from build123d import *

# Parameters (mm, degrees)
SKETCH1_W           = 28
SKETCH1_H           = 25
BOSS_EXTRUDE1_DEPTH = 2
SKETCH2_R           = 0.45
CUT_EXTRUDE1_DEPTH  = 10
SKETCH3_R           = 0.4
CUT_EXTRUDE2_DEPTH  = 2.5


with BuildPart() as part:
    # Sketch1 → Boss-Extrude1 (new body)
    with BuildSketch(Plane(origin=(0, 0, 0), x_dir=(1, 0, 0), z_dir=(0, 1, 0))):
        Rectangle(SKETCH1_W, SKETCH1_H)
    extrude(amount=BOSS_EXTRUDE1_DEPTH)

    # Sketch2 → Cut-Extrude1 (cut)
    with BuildSketch(Plane(origin=(0, 0, 0), x_dir=(1, 0, 0), z_dir=(0, 1, 0))):
        with Locations(Location((-9.52, -5.2, 0), (0, 0, 90))):
            Circle(SKETCH2_R)
        with Locations(Location((-9.52, -9.7, 0), (0, 0, 90))):
            Circle(SKETCH2_R)
    extrude(amount=CUT_EXTRUDE1_DEPTH, mode=Mode.SUBTRACT)

    # Sketch3 → Cut-Extrude2 (cut)
    with BuildSketch(Plane(origin=(0, 0, 0), x_dir=(1, 0, 0), z_dir=(0, 1, 0))):
        with Locations(Location((-11.13, 6.6, 0), (0, 0, 90))):
            Circle(SKETCH3_R)
        with Locations(Location((-11.13, 8.6, 0), (0, 0, 90))):
            Circle(SKETCH3_R)
        with Locations(Location((-11.13, 4.6, 0), (0, 0, 90))):
            Circle(SKETCH3_R)
    extrude(amount=CUT_EXTRUDE2_DEPTH, mode=Mode.SUBTRACT)


solid = part.part
Check sheet for the modelled part. Datum: model origin and axes. Units: mm. Round coordinates to 2 decimals unless told otherwise and drop trailing zeros. Write each loop counter-clockwise with the first axis right and the second up, starting at its lowest first coordinate (ties: lowest second). Pieces come first, ordered by that corner, then holes. Notation, with made-up numbers: (-9, 5.5) - (25, 5.5) arc R12 ccw to (25, 13.5) - close; hole circle Ø1 at (-3, -3.5). An arc over 180 degrees is marked (long way). Return JSON: item names as keys, results as strings.
Q1. Depth check by flat-ended pin: P1, Ø6, axis at x = -0.5, z = 7.5, coming from the -Y side. Enter the tip coordinate at first touch or a pass-through.
Returned:
{"P1": "stops at y = 0"}
Q2. Scan lines: L1, parallel to Z at x = -11.13, y = 1.65; L2, parallel to X at y = 0.95, z = 9.7; L3, parallel to X at y = 0.6, z = -8.6. Record each from-to range of solid material in increasing order. Write a range as from..to.
Returned:
{"L1": "z = -12.5..-9, -8.2..-7, -6.2..-5, -4.2..12.5", "L2": "x = -14..-9.97, -9.07..14", "L3": "x = -14..-11.53, -10.73..14"}
Q3. Cross-section at C-C (z = -8.6). Record the boundary of the cut face in (x, y), then the cut area to 3 significant figures.
Returned:
{"outline": "(-14, 0) - (-11.53, 0) - (-11.53, 2) - (-14, 2) - close; (-10.73, 0) - (14, 0) - (14, 2) - (-10.73, 2) - close", "area": "54.4 mm²"}
Q4. Cross-section at B-B (x = -9.52). Record the boundary of the cut face in (y, z), then the cut area to 3 significant figures.
Returned:
{"outline": "(0, -12.5) - (2, -12.5) - (2, 4.75) - (0, 4.75) - close; (0, 5.65) - (2, 5.65) - (2, 9.25) - (0, 9.25) - close; (0, 10.15) - (2, 10.15) - (2, 12.5) - (0, 12.5) - close", "area": "46.4 mm²"}
Q5. Draft check along X on faces 1 (the cylindrical face through (-9.966, 0.986, 5.259)), 2 (the flat face through (0, 1, -12.5)), 3 (the flat face through (-14, 1, 0)). Enter one of: released by +X, released by -X, zero draft, split by the parting line, or undercut.
Returned:
{"face 1": "undercut", "face 2": "zero draft", "face 3": "released by -X"}
Q6. Cross-section at A-A (z = 9.7). Record the boundary of the cut face in (x, y), then the cut area to 3 significant figures.
Returned:
{"outline": "(-14, 0) - (-9.97, 0) - (-9.97, 2) - (-14, 2) - close; (-9.07, 0) - (14, 0) - (14, 2) - (-9.07, 2) - close", "area": "54.2 mm²"}
